Geometry: final body of the model. Coordinates: model frame, mm. A direction names the side the tool comes from. Give positions to 0.01 mm unless a question says otherwise; leave off trailing zeros. Loops run counter-clockwise (first coordinate to the right, second up) from the corner with the lowest first, then second, coordinate; pieces in that order, holes last. Notation, with made-up numbers: (79.5, -13) -> (132.5, -13) arc R15 cw to (132.5, 6) -> close; hole circle Ø9 at (-24, 78). An arc over 180 degrees is marked (long way). One line per item, written item: value. Start each with the question number.
from build123d import *

# Parameters (mm, degrees)
F0_W      = 101.6
F0_H      = 177.8
F1_DEPTH  = 15.875
F1_FACE_W = 101.6
F1_FACE_H = 177.8
F2_DEPTH  = 15.875
F4_DEPTH  = 101.601
F5_W      = 12.7
F5_H      = 177.8
F6_DEPTH  = 9.525


with BuildPart() as f1:
    # F0 (on Top) → F1 (new body)
    with BuildSketch(Plane.XY):
        with Locations((-9.29141, -88.9)):
            Rectangle(F0_W, F0_H)
    extrude(amount=F1_DEPTH)

    # F1_face (on face) → F2 (join)
    with BuildSketch(Plane(origin=(-9.29141, -88.9, 0), x_dir=(1, 0, 0), z_dir=(0, 0, -1))):
        Rectangle(F1_FACE_W, F1_FACE_H)
    extrude(amount=F2_DEPTH)

    # F3 (on face) → F4 (cut, through all)
    with BuildSketch(Plane.YZ.offset(41.50859)):
        Polygon((-32.1183, -15.875), (-25.4, -15.875), (-25.4, -6.35), (-20.4343, -6.35), (-20.4343, 0.381), (-37.0967, 0.381), (-37.0967, -6.35), (-32.1183, -6.35), align=None)
        Polygon((-70.2183, -15.875), (-63.5, -15.875), (-63.5, -6.35), (-58.5343, -6.35), (-58.5343, 0.381), (-75.1967, 0.381), (-75.1967, -6.35), (-70.2183, -6.35), align=None)
        Polygon((-108.3183, -15.875), (-101.6, -15.875), (-101.6, -6.35), (-96.6343, -6.35), (-96.6343, 0.381), (-113.2967, 0.381), (-113.2967, -6.35), (-108.3183, -6.35), align=None)
        Polygon((-146.4183, -6.35), (-146.4183, -15.875), (-139.7, -15.875), (-139.7, -6.35), (-134.7343, -6.35), (-134.7343, 0.381), (-151.3967, 0.381), (-151.3967, -6.35), align=None)
    extrude(amount=-F4_DEPTH, mode=Mode.SUBTRACT)

    # F5 (on face) → F6 (join)
    with BuildSketch(Plane.XY.offset(15.875)):
        with Locations((-53.74141, -88.9)):
            Rectangle(F5_W, F5_H)
        with Locations((35.15859, -88.9)):
            Rectangle(F5_W, F5_H)
    extrude(amount=F6_DEPTH)


solid = f1.part
Item 1: Access query for faces 1 (the face through (-9, -151.397, -3)), 2 (the face through (-9, -108.318, -11)), 3 (the face through (-10, -13, -15.875)). Directions: +Z, -Z, +X, -X, +Y, -Y. A direction counts if a zero-diameter tool reaches every point of the face in a straight line with its end or side. Return the directions, or none.
Item 2: Section B-B, the plane y = -138. Output: boundary loops of the cut face in (x, z) (3 decimals), then the cut area to 3 significant figures.
Item 3: Section C-C, the plane z = -4. Output: boundary loops of the cut face in (x, y), then the cut area to 3 significant figures.
Item 4: Section A-A, the plane z = 21.5. Output: boundary loops of the cut face in (x, y).
Item 5: Pin query (flat end, axial travel): pin 1 (1.5 mm diameter, centred on x = 5, y = -98, fed in from +Z) (3 decimals); pin 2 (5 mm diameter, centred on x = -23, y = -66.5, fed in from -Z). Return the tip coordinate at first contact, or that it passes through.
Item 6: Mould query, pull axis Y, two halves, no side actions, for faces 4 (the face through (-9, -101.6, -11)), 5 (the face through (-10, 0, 0)), 6 (the face through (-10, -48, -15.875)). Classes: pulls with the +Y half, pulls with the -Y half, needs draft (parallel to the pull), parting line crosses it, or undercut.
Item 7: Ray query, line 1 along Y through (x, z) = (-21, -6); line 2 along Y through (x, z) = (-54.5, -12); line 3 along X through (y, z) = (-47, 23.5). Return the intervals inside material, ascending. Write a range as [from, to].
Geometry check:
1. face 1: +X, -X
1. face 2: -Z, +X, -X
1. face 3: -Z, +X, -X, +Y, -Y
2. outline: (-60.091, -15.875) -> (41.509, -15.875) -> (41.509, -6.35) -> (-60.091, -6.35) -> close; (-60.091, 0.381) -> (41.509, 0.381) -> (41.509, 25.4) -> (28.809, 25.4) -> (28.809, 15.875) -> (-47.391, 15.875) -> (-47.391, 25.4) -> (-60.091, 25.4) -> close
2. area: 2,780 mm2
3. outline: (-60.09, -177.8) -> (41.51, -177.8) -> (41.51, -151.4) -> (-60.09, -151.4) -> close; (-60.09, -134.73) -> (41.51, -134.73) -> (41.51, -113.3) -> (-60.09, -113.3) -> close; (-60.09, -96.63) -> (41.51, -96.63) -> (41.51, -75.2) -> (-60.09, -75.2) -> close; (-60.09, -58.53) -> (41.51, -58.53) -> (41.51, -37.1) -> (-60.09, -37.1) -> close; (-60.09, -20.43) -> (41.51, -20.43) -> (41.51, 0) -> (-60.09, 0) -> close
3. area: 11,300 mm2
4. outline: (-60.09, -177.8) -> (-47.39, -177.8) -> (-47.39, 0) -> (-60.09, 0) -> close; (28.81, -177.8) -> (41.51, -177.8) -> (41.51, 0) -> (28.81, 0) -> close
5. pin 1: stops at z = 15.875
5. pin 2: stops at z = 0.38
6. face 4: undercut
6. face 5: pulls with the +Y half
6. face 6: needs draft
7. line 1: y = [-177.8, -151.4], [-134.73, -113.3], [-96.63, -75.2], [-58.53, -37.1], [-20.43, 0]
7. line 2: y = [-177.8, -146.42], [-139.7, -108.32], [-101.6, -70.22], [-63.5, -32.12], [-25.4, 0]
7. line 3: x = [-60.09, -47.39], [28.81, 41.51]
